CAD build for the part. Positions are in the model's coordinates, mm. A direction names the side the tool comes from. Coordinates: 2 decimals unless noted, no trailing zeros. Loops run counter-clockwise (first coordinate to the right, second up) from the corner with the lowest first, then second, coordinate; pieces in that order, holes last. Notation, with made-up numbers: (-24, -11.5) -> (1, -11.5) arc R10 ccw to (1, 3.5) -> close; hole circle Ø10 at (26, 63.25). An arc over 180 degrees is marked (long way). Return JSON: item names as keys, results as strings. Group by question number.
(1) Tool access for faces 5 (the face through (0, -14.5, 11)), 6 (the face through (0, -17, 9)), 7 (the face through (14.5, 0, 7)): list every direction of +Z, -Z, +X, -X, +Y, -Y with a clear straight run to the whole face (end or side of a thin tool).
(2) Mould opens along Z. For faces 1 (the face through (-0.28, -9.27, 1.62)), 2 (the face through (-16.47, -12.03, 11.95)), 3 (the face through (16.47, -9.22, 12.2)), 4 (the face through (-4, 4, 0)) say: pulls with the +Z half, pulls with the -Z half, needs draft (parallel to the pull), parting line crosses it, or undercut.
(3) Saw through at C-C on y = 15. Write the cut outline in (x, z), then the cut area to 3 significant figures.
(4) Saw through at D-D on x = -15.5. Write the cut outline in (y, z).
(5) Flat gauge pin, fed straight in: pin 1 Ø2 at (x, y) = (-16.5, -0.5) entering from +Z. Where does the tip first touch, or does it go through?
(6) Saw through at A-A on x = 0. Give the number of separate pieces and of enclosed holes in the cut face, then the cut area to 3 significant figures.
(7) Probe L1, parallel to Y at x = 10, z = 1.6; L2, parallel to Y at x = 3, z = 10.75; L3, parallel to Z at x = 13.5, y = -16. List the from-to ranges inside material, lowest first.
(8) Saw through at B-B on z = 5.5. Write the cut outline in (x, y).
```python
from build123d import *

# Parameters (mm, degrees)
SKETCH_W        = 37
SKETCH_H        = 37
PAD_DEPTH       = 4
SKETCH001_W     = 4
SKETCH001_H     = 37
PAD001_DEPTH    = 10
SKETCH002_R     = 1.4
POCKET_DEPTH    = 100
POCKET003_DEPTH = 100
SKETCH004_R     = 1.3
SKETCH004_R_2   = 4.5
POCKET007_DEPTH = 5
SKETCH008_R     = 1.8
POCKET009_DEPTH = 10
CHAMFER_SIZE    = 1
CHAMFER001_SIZE = 0.2
SKETCH009_W     = 29
SKETCH009_H     = 4
PAD002_DEPTH    = 10
SKETCH010_W     = 29
SKETCH010_H     = 5
POCKET010_DEPTH = 100


with BuildPart() as part:
    # Sketch → Pad (new body)
    with BuildSketch(Plane.XY):
        Rectangle(SKETCH_W, SKETCH_H)
    extrude(amount=PAD_DEPTH)

    # Sketch001 (on Face6 of Pad) → Pad001 (join)
    with BuildSketch(Plane.XY.offset(4)):
        with Locations((16.5, 0)):
            Rectangle(SKETCH001_W, SKETCH001_H)
        with Locations((-16.5, 0)):
            Rectangle(SKETCH001_W, SKETCH001_H)
    extrude(amount=PAD001_DEPTH)

    # Sketch002 (on Face13 of Pad001) → Pocket (cut)
    with BuildSketch(Plane.YZ.offset(18.5)):
        with Locations((-11, 11)):
            Circle(SKETCH002_R)
        with Locations((11, 11)):
            Circle(SKETCH002_R)
    extrude(amount=-POCKET_DEPTH, mode=Mode.SUBTRACT)

    # Sketch006 → Pocket003 (cut)
    with BuildSketch(Plane(origin=(-20, 0, 0), x_dir=(0, -1, 0), z_dir=(-1, 0, 0))):
        with BuildLine():
            ThreePointArc((8, 10.650166), (0, 29.2), (-8, 10.650166))
            Line((-8, 10.650166), (-8, 7.2))
            Line((-8, 7.2), (8, 7.2))
            Line((8, 7.2), (8, 10.650166))
        make_face()
    extrude(amount=-POCKET003_DEPTH, mode=Mode.SUBTRACT)

    # Sketch004 → Pocket007 (cut)
    with BuildSketch(Plane.XY.offset(4)):
        with Locations((0, 8)):
            Circle(SKETCH004_R)
        with Locations((8, 0)):
            Circle(SKETCH004_R)
        with Locations((0, -8)):
            Circle(SKETCH004_R)
        with Locations((-8, 0)):
            Circle(SKETCH004_R)
        Circle(SKETCH004_R_2)
        with Locations((5.656854, 5.656854)):
            Circle(SKETCH004_R)
        with Locations((-5.656854, 5.656854)):
            Circle(SKETCH004_R)
        with Locations((-5.656854, -5.656854)):
            Circle(SKETCH004_R)
        with Locations((5.656854, -5.656854)):
            Circle(SKETCH004_R)
    extrude(amount=-POCKET007_DEPTH, mode=Mode.SUBTRACT)

    # Sketch008 → Pocket009 (cut)
    with BuildSketch(Plane(origin=(0, 0, 0), x_dir=(1, 0, 0), z_dir=(0, 0, -1))):
        with Locations((10, 10)):
            Circle(SKETCH008_R)
        with Locations((-10, 10)):
            Circle(SKETCH008_R)
        with Locations((-10, -10)):
            Circle(SKETCH008_R)
        with Locations((10, -10)):
            Circle(SKETCH008_R)
    extrude(amount=-POCKET009_DEPTH, mode=Mode.SUBTRACT)

    # Chamfer
    chamfer_edges = [part.edges().sort_by_distance(p)[0] for p in [
        (-6.956854, -5.656854, 4),
        (-1.3, -8, 4),
        (4.356854, -5.656854, 4),
        (6.7, 0, 4),
        (4.356854, 5.656854, 4),
        (-1.3, 8, 4),
        (-6.956854, 5.656854, 4),
        (-9.3, 0, 4),
    ]]
    chamfer(chamfer_edges, length=CHAMFER_SIZE)

    # Chamfer001
    chamfer001_edges = [part.edges().sort_by_distance(p)[0] for p in [
        (-6.956854, -5.656854, 0),
        (-9.3, 0, 0),
        (-6.956854, 5.656854, 0),
        (-1.3, 8, 0),
        (4.356854, 5.656854, 0),
        (6.7, 0, 0),
        (4.356854, -5.656854, 0),
        (-1.3, -8, 0),
        (-11.8, -10, 0),
        (-11.8, 10, 0),
        (8.2, 10, 0),
        (8.2, -10, 0),
    ]]
    chamfer(chamfer001_edges, length=CHAMFER001_SIZE)

    # Sketch009 (on Face3 of Chamfer001) → Pad002 (join)
    with BuildSketch(Plane.XY.offset(4)):
        with Locations((0, 16.5)):
            Rectangle(SKETCH009_W, SKETCH009_H)
        with Locations((0, -16.5)):
            Rectangle(SKETCH009_W, SKETCH009_H)
    extrude(amount=PAD002_DEPTH)

    # Sketch010 (on Face69 of Pad002) → Pocket010 (cut)
    with BuildSketch(Plane.XZ.offset(18.5)):
        with Locations((0, 6.5)):
            Rectangle(SKETCH010_W, SKETCH010_H)
    extrude(amount=-POCKET010_DEPTH, mode=Mode.SUBTRACT)


solid = part.part
```
Geometry results:
{
 "1": {"face 5": "+Z", "face 6": "+Y, -Y", "face 7": "none"},
 "2": {"face 1": "needs draft", "face 2": "undercut", "face 3": "pulls with the +Z half", "face 4": "pulls with the -Z half"},
 "3": {"outline": "(-18.5, 0) -> (18.5, 0) -> (18.5, 14) -> (-18.5, 14) -> close; hole (-14.5, 4) -> (14.5, 4) -> (14.5, 9) -> (-14.5, 9) -> close", "area": "373 mm²"},
 "4": {"outline": "(-18.5, 0) -> (18.5, 0) -> (18.5, 14) -> (10.17, 14) arc R11 cw to (8, 10.65) -> (8, 7.2) -> (-8, 7.2) -> (-8, 10.65) arc R11 cw to (-10.17, 14) -> (-18.5, 14) -> close; hole circle Ø2.8 at (-11, 11); hole circle Ø2.8 at (11, 11)"},
 "5": {"pin 1": "z = 7.2"},
 "6": {"separate pieces": "6", "enclosed holes": "0", "area": "129 mm²"},
 "7": {"L1": "-18.5 to -11.8, -8.2 to 8.2, 11.8 to 18.5", "L2": "-18.5 to -14.5, 14.5 to 18.5", "L3": "0 to 4, 9 to 14"},
 "8": {"outline": "(-18.5, -18.5) -> (-14.5, -18.5) -> (-14.5, 18.5) -> (-18.5, 18.5) -> close; (14.5, -18.5) -> (18.5, -18.5) -> (18.5, 18.5) -> (14.5, 18.5) -> close"}
}
